The listing builds one solid part. Answer for the finished solid, in the listing's coordinates (mm). A direction names the side the tool comes from. Coordinates: 2 decimals unless noted, no trailing zeros. Order: outer loops, then holes, each group sorted by start corner. A loop starts at its lowest first (then second) coordinate and runs counter-clockwise, first axis right, second up.
```python
from build123d import *

# Parameters (mm, degrees)
SKETCH1_W           = 60.452
SKETCH1_H           = 91.44
BOSS_EXTRUDE4_DEPTH = 2.54
SKETCH7_W           = 65.532
SKETCH7_H           = 96.52
SKETCH7_W_2         = 60.452
SKETCH7_H_2         = 91.44
BOSS_EXTRUDE5_DEPTH = 6.35
SKETCH8_R           = 1.651
BOSS_EXTRUDE6_DEPTH = 11.176
SKETCH10_W          = 60.452
SKETCH10_H          = 91.44
SKETCH10_W_2        = 56.896
SKETCH10_H_2        = 87.884
BOSS_EXTRUDE7_DEPTH = 3.048
SKETCH13_W          = 60.452
SKETCH13_H          = 91.44
SKETCH13_W_2        = 58.928
SKETCH13_H_2        = 89.916
BOSS_EXTRUDE8_DEPTH = 0.762
CUT_EXTRUDE1_REACH  = 61.923
SKETCH14_W          = 65.532
SKETCH14_H          = 96.52
SKETCH14_W_2        = 62.992
SKETCH14_H_2        = 93.98
FILLET1_R           = 5.08
FILLET3_R           = 0.508
FILLET4_R           = 0.508
FILLET5_R           = 1.016
SKETCH16_W          = 15.24
SKETCH16_H          = 15.24
SKETCH16_R          = 2.2479
BOSS_EXTRUDE9_DEPTH = 4.064
FILLET8_R           = 5.08


with BuildPart() as part:
    # Sketch1 → Boss-Extrude4 (new body)
    with BuildSketch(Plane(origin=(0, 0, 0), x_dir=(1, 0, 0), z_dir=(0, 1, 0))):
        Rectangle(SKETCH1_W, SKETCH1_H)
    extrude(amount=BOSS_EXTRUDE4_DEPTH)

    # Sketch7 → Boss-Extrude5 (add)
    with BuildSketch(Plane.XZ):
        Rectangle(SKETCH7_W, SKETCH7_H)
        Rectangle(SKETCH7_W_2, SKETCH7_H_2, mode=Mode.SUBTRACT)
    extrude(amount=-BOSS_EXTRUDE5_DEPTH)

    # Sketch8 → Boss-Extrude6 (add)
    with BuildSketch(Plane(origin=(0, 2.54, 0), x_dir=(1, 0, 0), z_dir=(0, 1, 0))):
        with Locations(Location((-24.13, 39.878, 0), (0, 0, 90))):
            Circle(SKETCH8_R)
        with Locations(Location((26.162, 39.878, 0), (0, 0, 90))):
            Circle(SKETCH8_R)
        with Locations(Location((-24.638, -41.402, 0), (0, 0, 90))):
            Circle(SKETCH8_R)
        with Locations(Location((25.908, -41.402, 0), (0, 0, 90))):
            Circle(SKETCH8_R)
    extrude(amount=BOSS_EXTRUDE6_DEPTH)

    # Sketch10 → Boss-Extrude7 (add)
    with BuildSketch(Plane(origin=(0, 2.54, 0), x_dir=(1, 0, 0), z_dir=(0, 1, 0))):
        Rectangle(SKETCH10_W, SKETCH10_H)
        Rectangle(SKETCH10_W_2, SKETCH10_H_2, mode=Mode.SUBTRACT)
    extrude(amount=BOSS_EXTRUDE7_DEPTH)

    # Sketch13 → Boss-Extrude8 (add)
    with BuildSketch(Plane(origin=(0, 5.588, 0), x_dir=(1, 0, 0), z_dir=(0, 1, 0))):
        Rectangle(SKETCH13_W, SKETCH13_H)
        Rectangle(SKETCH13_W_2, SKETCH13_H_2, mode=Mode.SUBTRACT)
    extrude(amount=BOSS_EXTRUDE8_DEPTH)

    # Sketch14 → Cut-Extrude1 (cut, up to next)
    with BuildSketch(Plane.XZ, mode=Mode.PRIVATE) as cut_extrude1_sk1:
        Rectangle(SKETCH14_W, SKETCH14_H)
        Rectangle(SKETCH14_W_2, SKETCH14_H_2, mode=Mode.SUBTRACT)
    cut_extrude1_tool1 = extrude(cut_extrude1_sk1.sketch, amount=-CUT_EXTRUDE1_REACH, mode=Mode.PRIVATE) & part.part
    add(cut_extrude1_tool1.solids().sort_by_distance((0, 0, -47.093357))[0], mode=Mode.SUBTRACT)

    # Fillet1
    fillet1_edges = [part.edges().sort_by_distance(p)[0] for p in [
        (-31.496, 3.175, -46.99),
        (-31.496, 3.175, 46.99),
        (31.496, 3.175, 46.99),
        (31.496, 3.175, -46.99),
    ]]
    fillet(fillet1_edges, radius=FILLET1_R)

    # Fillet3
    fillet3_edges = [part.edges().sort_by_distance(p)[0] for p in [
        (-24.13, 13.716, -38.227),
        (-24.638, 13.716, 43.053),
        (26.162, 13.716, -38.227),
        (25.908, 13.716, 43.053),
    ]]
    fillet(fillet3_edges, radius=FILLET3_R)

    # Fillet4
    fillet4_edges = [part.edges().sort_by_distance(p)[0] for p in [
        (29.464, 5.969, 44.958),
        (29.464, 5.969, -44.958),
        (-29.464, 5.969, -44.958),
        (-29.464, 5.969, 44.958),
    ]]
    fillet(fillet4_edges, radius=FILLET4_R)

    # Fillet5
    # the kernel refuses this fillet: 1.016 mm, written as the material it adds along each edge
    with BuildSketch(Plane(origin=(-27.432, 3.556, 42.926), x_dir=(-1, 0, 0), z_dir=(0, 0, 1))) as fillet5_piece_1_section:
        Polygon((0, 0), (FILLET5_R, 0), (FILLET5_R, FILLET5_R), (0, FILLET5_R), align=None)
    fillet5_piece_1 = extrude(amount=FILLET5_R, mode=Mode.PRIVATE)
    fillet5_piece_1 = fillet5_piece_1 - Plane(origin=(-27.432, 3.556, 42.926), x_dir=(0.7071067811865475, 0.7071067811865475, 0), z_dir=(0, 0, 1)) * Sphere(FILLET5_R, mode=Mode.PRIVATE)
    add(fillet5_piece_1)
    with BuildSketch(Plane(origin=(27.432, 3.556, 42.926), x_dir=(0, 0, 1), z_dir=(1, 0, 0))) as fillet5_piece_2_section:
        Polygon((0, 0), (FILLET5_R, 0), (FILLET5_R, FILLET5_R), (0, FILLET5_R), align=None)
    fillet5_piece_2 = extrude(amount=FILLET5_R, mode=Mode.PRIVATE)
    fillet5_piece_2 = fillet5_piece_2 - Plane(origin=(27.432, 3.556, 42.926), x_dir=(0, 0.7071067811865475, -0.7071067811865475), z_dir=(1, 0, 0)) * Sphere(FILLET5_R, mode=Mode.PRIVATE)
    add(fillet5_piece_2)
    with BuildSketch(Plane(origin=(27.432, 3.556, -42.926), x_dir=(0, 0, -1), z_dir=(1, 0, 0))) as fillet5_piece_3_section:
        Polygon((0, 0), (FILLET5_R, 0), (FILLET5_R, -FILLET5_R), (0, -FILLET5_R), align=None)
    fillet5_piece_3 = extrude(amount=FILLET5_R, mode=Mode.PRIVATE)
    fillet5_piece_3 = fillet5_piece_3 - Plane(origin=(27.432, 3.556, -42.926), x_dir=(0, 0.7071067811865475, 0.7071067811865475), z_dir=(1, 0, 0)) * Sphere(FILLET5_R, mode=Mode.PRIVATE)
    add(fillet5_piece_3)
    with BuildSketch(Plane(origin=(-27.432, 3.556, -42.926), x_dir=(-1, 0, 0), z_dir=(0, 0, -1))) as fillet5_piece_4_section:
        Polygon((0, 0), (FILLET5_R, 0), (FILLET5_R, -FILLET5_R), (0, -FILLET5_R), align=None)
    fillet5_piece_4 = extrude(amount=FILLET5_R, mode=Mode.PRIVATE)
    fillet5_piece_4 = fillet5_piece_4 - Plane(origin=(-27.432, 3.556, -42.926), x_dir=(0.7071067811865475, 0.7071067811865475, 0), z_dir=(0, 0, -1)) * Sphere(FILLET5_R, mode=Mode.PRIVATE)
    add(fillet5_piece_4)
    with BuildSketch(Plane(origin=(-27.432, 2.54, 43.942), x_dir=(0, 1, 0), z_dir=(1, 0, 0)), Plane(origin=(27.432, 2.54, -43.942), x_dir=(0, 1, 0), z_dir=(-1, 0, 0))) as fillet5_piece_5:
        with BuildLine():
            CenterArc((FILLET5_R, -FILLET5_R), FILLET5_R, 90, 90)
            Line((0, -FILLET5_R), (0, 0))
            Line((0, 0), (FILLET5_R, 0))
        make_face()
    extrude(amount=54.864)
    with BuildSketch(Plane(origin=(28.448, 2.54, 42.926), x_dir=(0, 1, 0), z_dir=(0, 0, -1)), Plane(origin=(-28.448, 2.54, -42.926), x_dir=(0, 1, 0), z_dir=(0, 0, 1))) as fillet5_piece_6:
        with BuildLine():
            CenterArc((FILLET5_R, -FILLET5_R), FILLET5_R, 90, 90)
            Line((0, -FILLET5_R), (0, 0))
            Line((0, 0), (FILLET5_R, 0))
        make_face()
    extrude(amount=85.852)
    with BuildSketch(Plane(origin=(28.448, 3.556, 43.942), x_dir=(0, 0, -1), z_dir=(0, 1, 0)), Plane(origin=(-28.448, 3.556, 43.942), x_dir=(1, 0, 0), z_dir=(0, 1, 0))) as fillet5_piece_7:
        with BuildLine():
            CenterArc((FILLET5_R, FILLET5_R), FILLET5_R, 180, 90)
            Line((0, FILLET5_R), (0, 0))
            Line((0, 0), (FILLET5_R, 0))
        make_face()
    extrude(amount=2.032)
    with BuildSketch(Plane(origin=(28.448, 3.556, -43.942), x_dir=(0, 0, 1), z_dir=(0, 1, 0)), Plane(origin=(-28.448, 3.556, -43.942), x_dir=(1, 0, 0), z_dir=(0, 1, 0))) as fillet5_piece_8:
        with BuildLine():
            CenterArc((FILLET5_R, -FILLET5_R), FILLET5_R, 90, 90)
            Line((0, -FILLET5_R), (0, 0))
            Line((0, 0), (FILLET5_R, 0))
        make_face()
    extrude(amount=2.032)

    # Sketch16 → Boss-Extrude9 (add)
    # profile 1 of 2: a face of its own
    with BuildSketch(Plane.XZ):
        with Locations((0.031289089, 54.61)):
            Rectangle(SKETCH16_W, SKETCH16_H)
        with Locations(Location((0, 54.61, 0), (0, 0, 270))):
            Circle(SKETCH16_R, mode=Mode.SUBTRACT)
    # profile 2 of 2: a face of its own
    with BuildSketch(Plane.XZ):
        Polygon((7.62, -46.99), (0, -46.99), (-7.62, -46.99), (-7.62, -62.23), (7.62, -62.23), align=None)
        with Locations(Location((0, -54.61, 0), (0, 0, 270))):
            Circle(SKETCH16_R, mode=Mode.SUBTRACT)
    extrude(amount=-BOSS_EXTRUDE9_DEPTH)

    # Fillet8
    fillet8_edges = [part.edges().sort_by_distance(p)[0] for p in [
        (7.651289089, 2.032, 62.23),
        (7.651289089, 2.032, 46.99),
        (-7.588710911, 2.032, 46.99),
        (-7.588710911, 2.032, 62.23),
        (7.62, 2.032, -46.99),
        (7.62, 2.032, -62.23),
        (-7.62, 2.032, -62.23),
        (-7.62, 2.032, -46.99),
    ]]
    fillet(fillet8_edges, radius=FILLET8_R)


solid = part.part
```
1) A cutting plane is placed at A-A, the plane x = 0. Write down the section's boundary in (y, z), plus the area to 3 significant figures.
2) The mould has two halves that part along Z. Classify faces 4 (the flat face through (0, 2.54, -1)), 5 (the flat face through (26, 13.716, -40)), 6 (the cylindrical face through (6.171, 2.06, -60.702)), 7 (the cylindrical face through (30.05, 3.22, 45.46)): released by +Z, released by -Z, zero draft, split by the parting line, or undercut.
3) A cutting plane is placed at D-D, the plane z = 19. Write down the section's boundary in (x, y), plus the area to 3 significant figures.
4) Each of these flat-tipped pins is pushed along its axis until it touches: P1, Ø4.5, axis at y = 2, z = 55, coming from the +X side; P2, Ø10, axis at x = -6, z = 24, coming from the +Y side; P3, Ø1.2, axis at y = 1.5, z = -54, coming from the +X side. Where does it stop, or does it pass through?
5) For faces 1 (the flat face through (29, 5.588, 0)), 2 (the flat face through (-7.62, 2, -55)), 3 (the flat face through (-25, 13.716, 41)), determine the directions among +Z, -Z, +X, -X, +Y, -Y from which every point of the face is accessible in a straight line to the end or side of a thin tool.
6) A cutting plane is placed at C-C, the plane x = -18.5. Write down the section's boundary in (y, z).
7) A cutting plane is placed at B-B, the plane z = -54.61. Write down the section's boundary in (x, y).
8) Straight lines are drawn through the part: probe 1 along X at (y, z) = (1.5, 54.61); probe 2 along X at (y, z) = (1.7, -54.61); probe 3 along Z at (x, y) = (8, 5.75). For each, find the intervals that lie inside material, in ascending order.
Working result:
1. outline: (0, -62.23) - (4.06, -62.23) - (4.06, -56.86) - (0, -56.86) - close; (0, -52.36) - (4.06, -52.36) - (4.06, -46.99) - (6.35, -46.99) - (6.35, -44.96) - (5.59, -44.96) - (5.59, -43.94) - (3.56, -43.94) arc R1.02 cw to (2.54, -42.93) - (2.54, 42.93) arc R1.02 cw to (3.56, 43.94) - (5.59, 43.94) - (5.59, 44.96) - (6.35, 44.96) - (6.35, 46.99) - (4.06, 46.99) - (4.06, 52.36) - (0, 52.36) - close; (0, 56.86) - (4.06, 56.86) - (4.06, 62.23) - (0, 62.23) - close
1. area: 348 mm2
2. face 4: undercut
2. face 5: zero draft
2. face 6: released by -Z
2. face 7: released by +Z
3. outline: (-31.5, 0) - (31.5, 0) - (31.5, 6.35) - (29.46, 6.35) - (29.46, 5.59) - (28.45, 5.59) - (28.45, 3.56) arc R1.02 cw to (27.43, 2.54) - (-27.43, 2.54) arc R1.02 cw to (-28.45, 3.56) - (-28.45, 5.59) - (-29.46, 5.59) - (-29.46, 6.35) - (-31.5, 6.35) - close
3. area: 182 mm2
4. P1: stops at x = 7.65
4. P2: stops at y = 2.54
4. P3: stops at x = 7.62
5. face 1: +Y
5. face 2: -Z, -X, +Y, -Y
5. face 3: +Z, -Z, +X, -X, +Y
6. outline: (0, -46.99) - (6.35, -46.99) - (6.35, -44.96) - (5.59, -44.96) - (5.59, -43.94) - (3.56, -43.94) arc R1.02 cw to (2.54, -42.93) - (2.54, 42.93) arc R1.02 cw to (3.56, 43.94) - (5.59, 43.94) - (5.59, 44.96) - (6.35, 44.96) - (6.35, 46.99) - (0, 46.99) - close
7. outline: (-7.62, 0) - (-2.25, 0) - (-2.25, 4.06) - (-7.62, 4.06) - close; (2.25, 0) - (7.62, 0) - (7.62, 4.06) - (2.25, 4.06) - close
8. probe 1: x = -7.59 to -2.25, 2.25 to 7.65
8. probe 2: x = -7.62 to -2.25, 2.25 to 7.62
8. probe 3: z = -46.99 to -44.96, 44.96 to 46.99
